Geometry check sheet. Reference: the model listing, model coordinates, mm. Face numbers are marked on the shaded views. Give positions to 0.01 mm unless a question says otherwise; leave off trailing zeros. Write each loop counter-clockwise with the first axis right and the second up, starting at its lowest first coordinate (ties: lowest second). Pieces come first, ordered by that corner, then holes. Notation, with made-up numbers: M 53.25,-15 L 92.25,-15 A29 ccw 92.25,11 Z; hole C -7,-0.5 d8. An arc over 180 degrees is marked long. One line per item, written item: value. Start each with the question number.
1. Cross-section at C-C on y = 77. Record the cut outline in (x, z) (3 decimals).
2. Cross-section at B-B on x = 128.5. Record the cut outline in (y, z).
3. Cross-section at A-A on z = 8. Record the cut outline in (x, y) (3 decimals).
4. Scan lines: line 1 (Y direction, x = 74.5, z = 10); line 2 (X direction, y = 5, z = 5.75) (3 decimals); line 3 (Z direction, x = 230, y = 120.5). Record each from-to range of solid material in increasing order.
5. Release check for a two-part mould opening along Y. For the marked faces 1, 2, 3 and 4 record: pulls with the +Y half, pulls with the -Y half, needs draft (parallel to the pull), parting line crosses it, or undercut.
6. Gauge pin test, flat end, axial feed: pin 1 (1 mm diameter, centred on x = 124, y = 27, fed in from +Z). Record the tip position at first contact, or that the pin passes through.
Autodesk Fusion 360 part; units mm, degrees
sketch "Sketch1" plane through (0, 0, 0) normal (0, 0, 1) x (1, 0, 0)
  line L0 (0, 0) -> (350.815, 0)
  line L1 (350.815, 0) -> (350.815, 124.629)
  line L2 (0, 124.629) -> (0, 0)
  line L3 (350.815, 0) -> (350.815, 124.629)
  line L4 (344.815, 129.629) -> (0, 129.629)
  line L5 (0, 0) -> (0, 124.629)
  line L6 (0, 0) -> (350.815, 0)
  line L7 (0, 129.629) -> (344.815, 129.629)
  line L8 (350.815, 124.629) -> (0, 124.629)
  line L9 (350.815, 124.629) -> (350.815, 0)
  line L10 (355.815, 6) -> (355.815, 118.629)
  line L11 (344.815, -5) -> (6, -5)
  line L12 (-5, -5) -> (-5, 0)
  line L13 (0, 0) -> (350.815, 0)
  line L14 (0, 0) -> (0, 124.629)
  line L15 (0, 129.629) -> (6, 129.629)
  line L16 (-5, 118.629) -> (-5, 6)
  arc A0 (-5, 6) -> (6, -5) centre (6, 6) ccw
  arc A1 (6, 129.629) -> (-5, 118.629) centre (6, 118.629) ccw
  arc A2 (344.815, -5) -> (355.815, 6) centre (344.815, 6) ccw
  arc A3 (355.815, 118.629) -> (344.815, 129.629) centre (344.815, 118.629) ccw
  line L17 (6, 129.629) -> (0, 129.629)
  point P0 (355.815, 129.629)
  point P1 (355.815, -5)
  dimension "d12" = 355.815
  dimension "d13" = 5
  dimension "d16" = 11
  dimension "d17" = 11
  dimension "d18" = 11
  dimension "d19" = 11
  dimension "d24" = 360.815
  dimension "d25" = 134.629
extrude "Extrude1" add sketch "Sketch1" along normal blind 3 contours L0 L1 L2 L3 L5 L6 L8 L9 L13 L14
extrude "Extrude2" add sketch "Sketch1" along normal blind 25
equation "d12 = 350.815 mm + 5 mm"
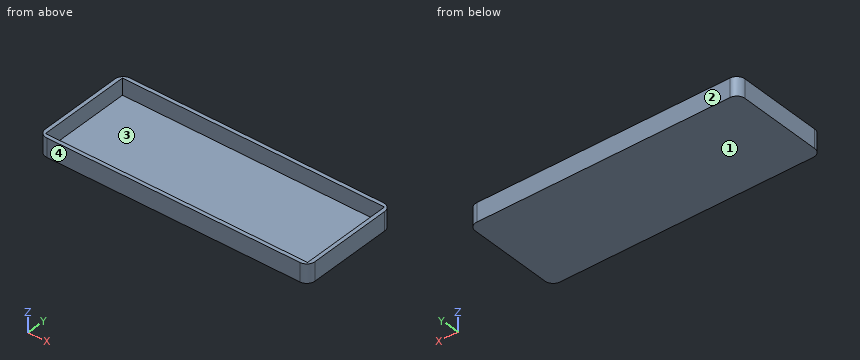
Report:
1. outline: M -5,0 L 355.815,0 L 355.815,25 L 350.815,25 L 350.815,3 L 0,3 L 0,25 L -5,25 Z
2. outline: M -5,0 L 129.63,0 L 129.63,25 L 124.63,25 L 124.63,3 L 0,3 L 0,25 L -5,25 Z
3. outline: M -5,6 A11 ccw 6,-5 L 344.815,-5 A11 ccw 355.815,6 L 355.815,118.629 A11 ccw 344.815,129.629 L 6,129.629 A11 ccw -5,118.629 Z; hole M 0,0 L 350.815,0 L 350.815,124.629 L 0,124.629 Z
4. line 1: y = -5 to 0, 124.63 to 129.63
4. line 2: x = -4.954 to 0, 350.815 to 355.769
4. line 3: z = 0 to 3
5. face 1: needs draft
5. face 2: pulls with the +Y half
5. face 3: undercut
5. face 4: pulls with the -Y half
6. pin 1: stops at z = 3
